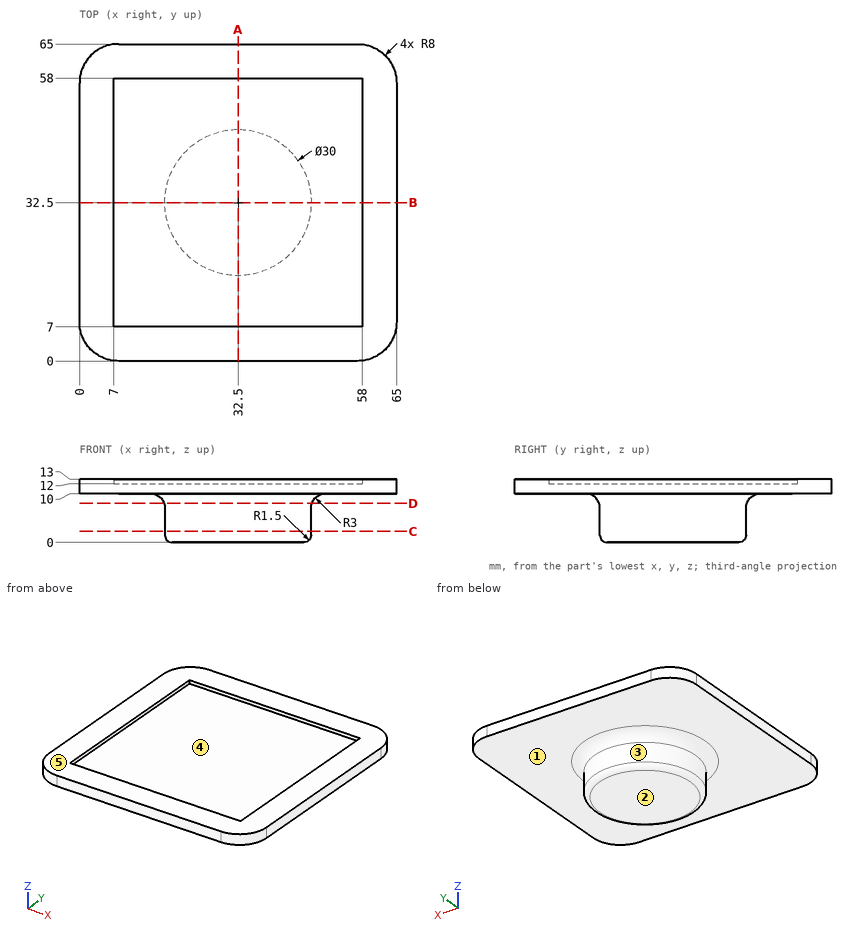
Answer from the drawing. Dimensions are ordinates in mm from the lowest x, y and z of the part. A direction names the side the tool comes from. Coordinates: 2 decimals unless noted, no trailing zeros. Order: outer loops, then holes, each group sorted by start corner. A loop starts at its lowest first (then second) coordinate and runs counter-clockwise, first axis right, second up. Notation, with made-up numbers: M -17.75,86 L 30.25,86 A18 ccw 30.25,92 Z; hole C 10.5,-24.5 d7. An arc over 180 degrees is marked long. Put each result on its own line as item: value. Start each with the question number.
Item 1: Given pin 1 Ø1.5 at (x, z) = (32.5, 5.5) entering from -Y; pin 2 Ø12 at (x, y) = (11, 13.5) entering from +Z; pin 3 Ø2 at (y, z) = (47, 5.5) entering from -X; pin 4 Ø6 at (y, z) = (36, 5) entering from -X, each flat-ended and moving along its own axis, determine where each tip first touches the part or whether it passes through.
Item 2: Section A-A, the plane x = 32.5 is taken. Determine the outline of the cut face in (y, z), plus the area to 3 significant figures.
Item 3: Consider probe 1 along Y at (x, z) = (56.5, 12.25); probe 2 along Z at (x, y) = (40.5, 60). Determine where each line is inside the solid, lowest interval first. Write a range as [from, to].
Item 4: The mould has two halves that part along X. Classify the marked faces 3, 4 and 5: +X half, -X half, draft (parallel to the pull), parting line (faces both ways), or undercut.
Item 5: For the marked faces 1 and 2, determine the directions among +Z, -Z, +X, -X, +Y, -Y from which every point of the face is accessible in a straight line to the end or side of a thin tool.
Item 6: Section D-D, the plane z = 8 is taken. Determine the outline of the cut face in (x, y).
Item 7: Section C-C, the plane z = 2.25 is taken. Determine the outline of the cut face in (x, y).
Computed:
1. pin 1: stops at y = 17.5
1. pin 2: stops at z = 13
1. pin 3: stops at x = 25.96
1. pin 4: stops at x = 17.51
2. outline: M 0,10 L 14.5,10 A3 cw 17.5,7 L 17.5,1.5 A1.5 ccw 19,0 L 46,0 A1.5 ccw 47.5,1.5 L 47.5,7 A3 cw 50.5,10 L 65,10 L 65,13 L 58,13 L 58,12 L 7,12 L 7,13 L 0,13 Z
2. area: 447 mm2
3. probe 1: y = [0, 7], [58, 65]
3. probe 2: z = [10, 13]
4. face 3: parting line
4. face 4: undercut
4. face 5: draft
5. face 1: -Z
5. face 2: -Z, +X, -X, +Y, -Y
6. outline: C 32.5,32.5 d30.34
7. outline: C 32.5,32.5 d30
